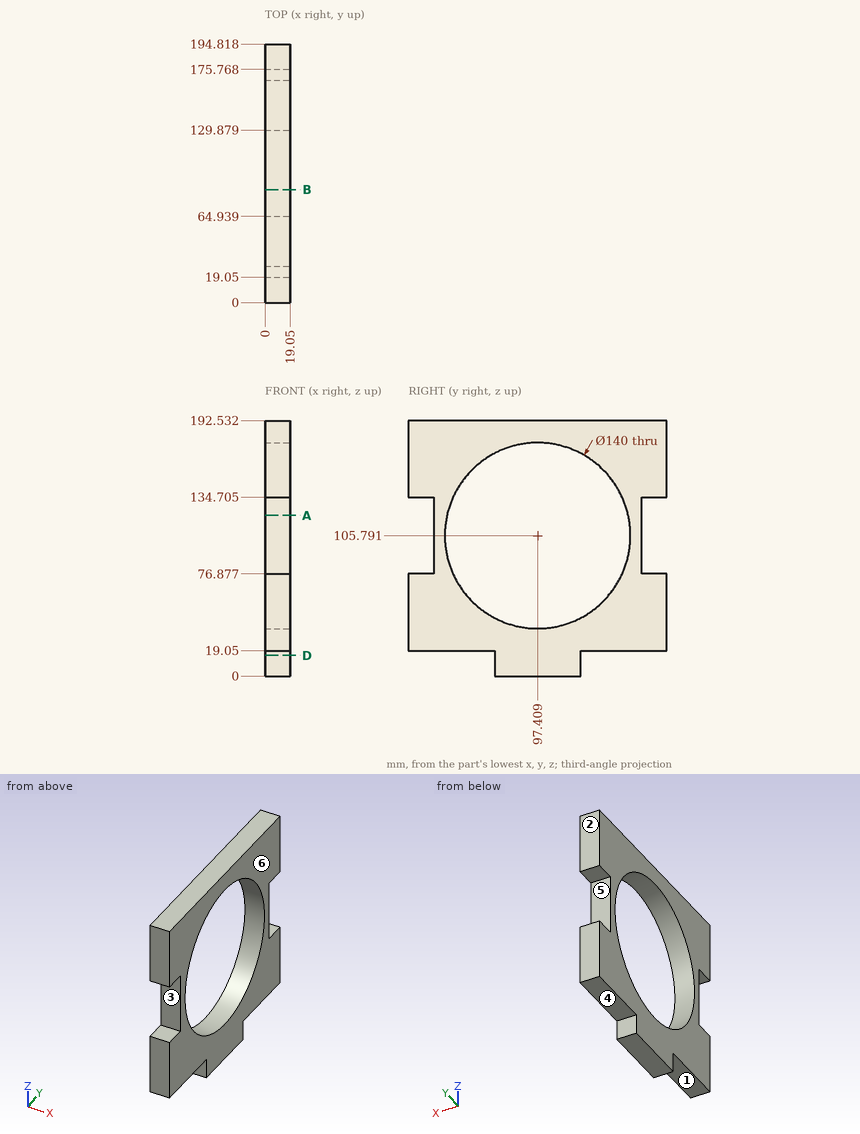
Check sheet for the drawn part. Datum: minimum x, y, z corner. Units: mm. A direction names the side the tool comes from. Give positions to 0.01 mm unless a question says otherwise; leave off trailing zeros. Write each loop counter-clockwise with the first axis right and the second up, starting at its lowest first coordinate (ties: lowest second). Pieces come first, ordered by that corner, then holes. Notation, with made-up numbers: M 76.5,84 L 130.5,84 A30 cw 130.5,106 Z; hole C 77.25,-24.5 d3. An arc over 180 degrees is marked long. Write item = value, one per line.
(1) Go/stop test with flat-tipped pins: pin 1 Ø8 at (x, y) = (11.5, 52.5) entering from -Z; pin 2 Ø9.5 at (x, z) = (6, 9.5) entering from -Y; pin 3 Ø5.5 at (x, z) = (13.5, 106.5) entering from +Y. Record where each tip stops, or that it passes through.
Found:
pin_1 = 19.05
pin_2 = 64.94
pin_3 = 175.77
(2) Sectioned sample at A-A (z = 121). Record the cut outline in (x, y), then the cut area to 3 significant figures.
Found:
outline = M 0,19.05 L 19.05,19.05 L 19.05,29.08 L 0,29.08 Z; M 0,165.74 L 19.05,165.74 L 19.05,175.77 L 0,175.77 Z
area = 382 mm2
(3) Access from +Z, -Z, +X, -X, +Y, -Y to the whole of each face (thin tool, end or side, straight path). Record for the marked faces 4, 5 and 6.
Found:
face_4 = -Z, +X, -X, +Y
face_5 = +X, -X, +Y
face_6 = +Z, -Z, +X, +Y, -Y
(4) Draft check along Z on the marked faces 1, 2 and 3. Enter one of: released by +Z, released by -Z, zero draft, split by the parting line, or undercut.
Found:
face_1 = released by -Z
face_2 = zero draft
face_3 = undercut
(5) Material ranges on line 1 (Z direction, x = 2.75, y = 98); line 2 (Z direction, x = 1, y = 172.5); line 3 (Z direction, x = 3.75, y = 74), recorded low to high.
Found:
line_1 = 0 to 35.79, 175.79 to 192.53
line_2 = 19.05 to 192.53
line_3 = 0 to 39.82, 171.76 to 192.53
(6) Sectioned sample at D-D (z = 15.5). Record the cut outline in (x, y).
Found:
outline = M 0,64.94 L 19.05,64.94 L 19.05,129.88 L 0,129.88 Z
(7) Sectioned sample at B-B (y = 85). Record the cut outline in (x, z), then the cut area to 3 significant figures.
Found:
outline = M 0,0 L 19.05,0 L 19.05,36.9 L 0,36.9 Z; M 0,174.68 L 19.05,174.68 L 19.05,192.53 L 0,192.53 Z
area = 1,040 mm2
